Verification items for this drawing (mm, ordinates from the low corner). Round coordinates to 2 decimals unless told otherwise and drop trailing zeros. Order: outer loops, then holes, each group sorted by start corner. A loop starts at its lowest first (then second) coordinate and runs counter-clockwise, first axis right, second up. Notation, with made-up numbers: (-9, 83) - (9, 83) arc R29 ccw to (9, 105) - close; hole circle Ø6 at (-19.5, 0). An arc over 180 degrees is marked (long way). Use a Markdown table: item, result. Add a question column.
(1) Section check A-A on y = 2.75. Record the boundary of the cut face in (x, z).
(2) Thickness scan on line 1 along X through (y, z) = (1.75, 177.8); line 2 along Z through (x, y) = (177.8, 1.5); line 3 along X through (y, z) = (3.25, 104.5). Record the ranges inside material, lowest first. Write a range as [from, to].
(3) Section check C-C on x = 152.4. Record the boundary of the cut face in (y, z), then the cut area to 3 significant figures.
(4) Section check B-B on z = 25.4. Record the boundary of the cut face in (x, y), then the cut area to 3 significant figures.
(5) Section check D-D on z = 135.5. Record the boundary of the cut face in (x, y).
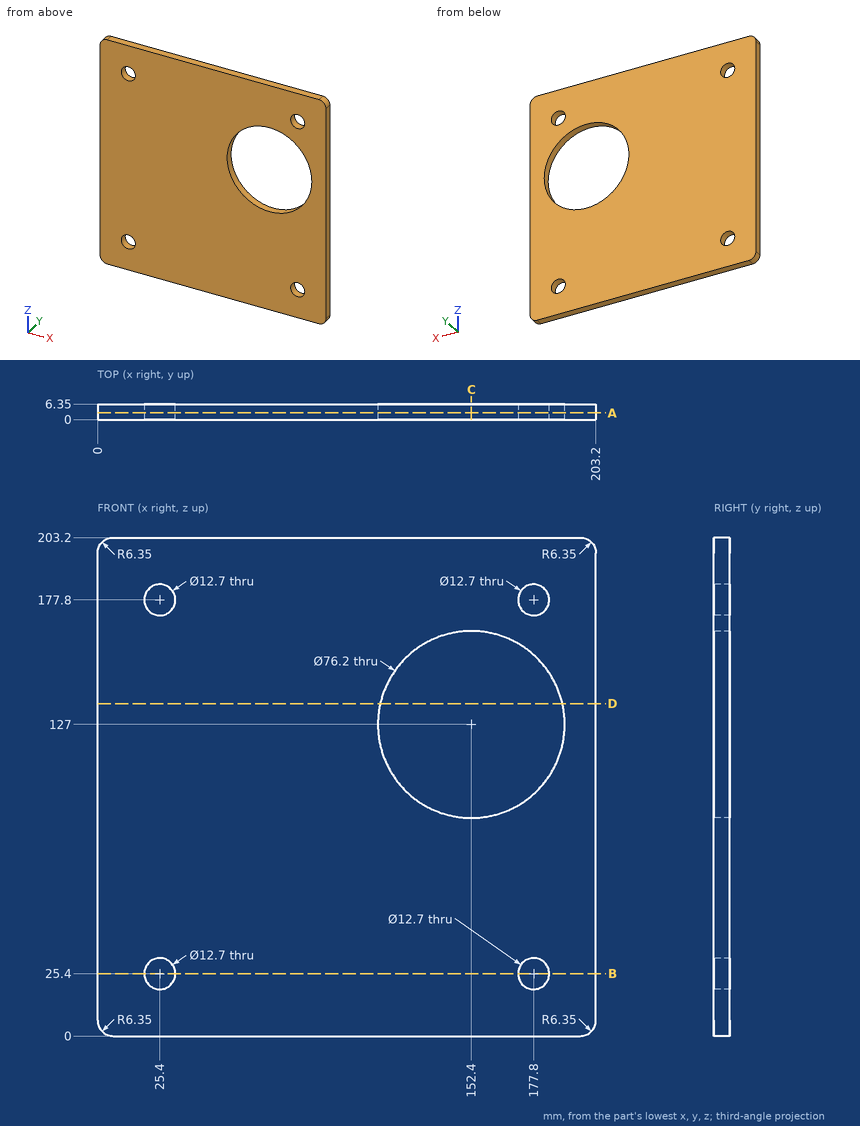
Check sheet entries:
| question | item | result |
|---|---|---|
| 1 | outline | (0, 6.35) arc R6.35 ccw to (6.35, 0) - (196.85, 0) arc R6.35 ccw to (203.2, 6.35) - (203.2, 196.85) arc R6.35 ccw to (196.85, 203.2) - (6.35, 203.2) arc R6.35 ccw to (0, 196.85) - close; hole circle Ø12.7 at (25.4, 25.4); hole circle Ø12.7 at (25.4, 177.8); hole circle Ø76.2 at (152.4, 127); hole circle Ø12.7 at (177.8, 25.4); hole circle Ø12.7 at (177.8, 177.8) |
| 2 | line 1 | x = [0, 19.05], [31.75, 171.45], [184.15, 203.2] |
| 2 | line 2 | z = [0, 19.05], [31.75, 98.6], [155.4, 171.45], [184.15, 203.2] |
| 2 | line 3 | x = [0, 121.65], [183.15, 203.2] |
| 3 | outline | (0, 0) - (6.35, 0) - (6.35, 88.9) - (0, 88.9) - close; (0, 165.1) - (6.35, 165.1) - (6.35, 203.2) - (0, 203.2) - close |
| 3 | area | 806 mm2 |
| 4 | outline | (0, 0) - (19.05, 0) - (19.05, 6.35) - (0, 6.35) - close; (31.75, 0) - (171.45, 0) - (171.45, 6.35) - (31.75, 6.35) - close; (184.15, 0) - (203.2, 0) - (203.2, 6.35) - (184.15, 6.35) - close |
| 4 | area | 1,130 mm2 |
| 5 | outline | (0, 0) - (115.26, 0) - (115.26, 6.35) - (0, 6.35) - close; (189.54, 0) - (203.2, 0) - (203.2, 6.35) - (189.54, 6.35) - close |
